from build123d import *

# Parameters (mm, degrees)
SKETCH1_R               = 40
BOSS_EXTRUDE1_DEPTH     = 20
FILLET1_R               = 10
SHELL1_T                = -2
CUT_EXTRUDE1_DEPTH      = 61.000000133
CUT_EXTRUDE1_DEPTH_BACK = 61.000000133


with BuildPart() as part:
    # Sketch1 → Boss-Extrude1 (new body)
    with BuildSketch(Plane(origin=(0, 0, 0), x_dir=(1, 0, 0), z_dir=(0, 1, 0))):
        with Locations(Location((0, 0, 0), (0, 0, 270))):
            Circle(SKETCH1_R)
    extrude(amount=BOSS_EXTRUDE1_DEPTH)

    # Fillet1
    fillet1_edges = [part.edges().sort_by_distance(p)[0] for p in [
        (0, 0, -40),
    ]]
    fillet(fillet1_edges, radius=FILLET1_R)

    # Shell1
    shell1_openings = [part.faces().sort_by_distance(p)[0] for p in [
        (0, 20, 0),
    ]]
    offset(amount=SHELL1_T, openings=shell1_openings, kind=Kind.INTERSECTION)

    # Sketch2 → Cut-Extrude1 (cut, two sides: drawn at the far end of the back side and taken through both)
    with BuildSketch(Plane.XY.offset(-CUT_EXTRUDE1_DEPTH_BACK)):
        Polygon((-17.458737084, 27.458737084), (0, 10), (20.279769331, 30.279769331), align=None)
    extrude(amount=CUT_EXTRUDE1_DEPTH + CUT_EXTRUDE1_DEPTH_BACK, mode=Mode.SUBTRACT)


solid = part.part
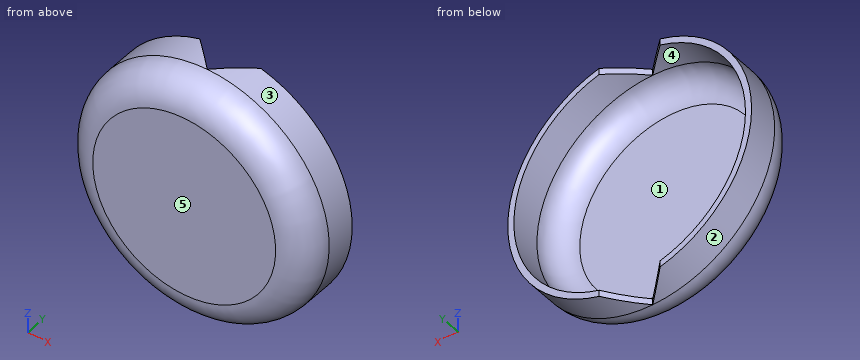
Geometry: final body of the model. Coordinates: model frame, mm. Face numbers are marked on the shaded views. A direction names the side the tool comes from. Round coordinates to 2 decimals unless told otherwise and drop trailing zeros. Order: outer loops, then holes, each group sorted by start corner. A loop starts at its lowest first (then second) coordinate and runs counter-clockwise, first axis right, second up. Notation, with made-up numbers: (-34, -33) - (-22, -33) arc R23 cw to (-22, -25) - close; hole circle Ø2 at (35, 24). An arc over 180 degrees is marked (long way). Write each question's results on one line, items separated by ' | '.
Item 1: Section B-B, the plane z = 0. Return the cut outline in (x, y), and give its area (3 significant figures).
Completed:
outline: (-40, 10) arc R10 ccw to (-30, 0) - (30, 0) arc R10 ccw to (40, 10) - (40, 20) - (38, 20) - (38, 10) arc R8 cw to (30, 2) - (-30, 2) arc R8 cw to (-38, 10) - (-38, 20) - (-40, 20) - close | area: 217 mm^2
Item 2: Section A-A, the plane y = 17.25. Return the cut outline in (x, z).
Completed:
outline: (-7.25, -39.34) - (-7.25, -37.3) arc R38 cw to (-7.25, 37.3) - (-7.25, 39.34) arc R40 ccw to start; (7.25, -39.34) arc R40 ccw to (7.25, 39.34) - (7.25, 37.3) arc R38 cw to (7.25, -37.3) - close
Item 3: Mould query, pull axis Z, two halves, no side actions, for the marked faces 3, 4 and 5. Classes: pulls with the +Z half, pulls with the -Z half, needs draft (parallel to the pull), parting line crosses it, or undercut.
Completed:
face 3: parting line crosses it | face 4: undercut | face 5: needs draft
Item 4: Reachability of the marked faces 1 and 2 from +Z, -Z, +X, -X, +Y, -Y: full face, straight path, thin tool, end or side. Return the list, or none.
Completed:
face 1: +Y | face 2: -X, +Y, -Y
Item 5: Section D-D, the plane y = 3.5. Return the cut outline in (x, z), and give its area (3 significant figures).
Completed:
outline: circle Ø75.2 at (0, 0); hole circle Ø69.33 at (0, 0) | area: 666 mm^2
Item 6: Material intervals for line 1 along Y through (x, z) = (-2.5, 2.5); line 2 along X through (y, z) = (10.5, 3.5); line 3 along X through (y, z) = (16.25, 23), sorted ascending. Write a range as [from, to].
Completed:
line 1: [0, 2] | line 2: [-39.85, -37.84], [37.84, 39.85] | line 3: [-32.73, -30.25], [30.25, 32.73]
Item 7: First-contact query: pin 1 Ø4 at (y, z) = (10.5, -12.5) entering from +X; pin 2 Ø2 at (x, z) = (-2.5, -30) entering from +Y; pin 3 Ø4 at (x, y) = (8, 16) entering from +Z; pin 4 Ø4 at (x, z) = (-7, 6.5) entering from -Y. Flat tips, straight axial feed; report the tip coordinate or a pass-through.
Completed:
pin 1: x = 38.6 | pin 2: y = 2.08 | pin 3: z = 39.55 | pin 4: y = 0
